For this review, take the finished solid that the model builds, in its own axes (mm). Face numbers are marked on the shaded views. A direction names the side the tool comes from. Coordinates: 2 decimals unless noted, no trailing zeros. Order: outer loops, then holes, each group sorted by start corner. A loop starts at its lowest first (then second) coordinate and runs counter-clockwise, first axis right, second up. Notation, with made-up numbers: M 46,57 L 66,57 A22 cw 66,94 Z; hole C 88.25,-32.5 d2. An arc over 180 degrees is marked long. Use CSV: the item, a comma, the result in double quotes.
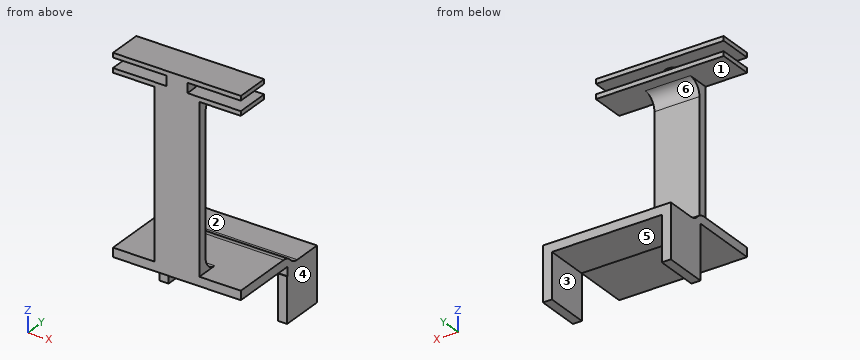
```python
from build123d import *

# Parameters (mm, degrees)
ESQUISSE1_W                = 28.4
ESQUISSE1_H                = 15.1
BOSS_EXTRU_1_DEPTH         = 2
ESQUISSE2_W                = 28.4
ESQUISSE2_H                = 9.6
BOSS_EXTRU_2_DEPTH         = 2
ESQUISSE3_W                = 2
ESQUISSE3_H                = 9.6
ESQUISSE3_H_2              = 9.7
BOSS_EXTRU_3_DEPTH         = 10
ESQUISSE4_W                = 10
ESQUISSE4_H                = 40
BOSS_EXTRU_4_DEPTH         = 2
BOSS_EXTRU_5_DEPTH         = 2.2
ESQUISSE6_W                = 28.4
ESQUISSE6_H                = 7.560696408
BOSS_EXTRU_6_DEPTH         = 1
R_P_TITION_LIN_AIRE1_COUNT = 2
R_P_TITION_LIN_AIRE1_PITCH = 3.2
ESQUISSE7_W                = 2.65
ESQUISSE7_H                = 2.2
ENL_V_MAT_EXTRU_1_DEPTH    = 57.310301011
BOSS_EXTRU_7_DEPTH         = 28.4
CONG_1_R                   = 3


with BuildPart() as part:
    # Esquisse1 → Boss.-Extru.1 (new body)
    with BuildSketch(Plane.XY):
        with Locations((14.2, 7.55)):
            Rectangle(ESQUISSE1_W, ESQUISSE1_H)
    extrude(amount=BOSS_EXTRU_1_DEPTH)

    # Esquisse4 → Boss.-Extru.4 (add)
    with BuildSketch(Plane.XZ):
        with Locations((14.2, 22)):
            Rectangle(ESQUISSE4_W, ESQUISSE4_H)
    extrude(amount=-BOSS_EXTRU_4_DEPTH)

    # Esquisse5 → Boss.-Extru.5 (add)
    with BuildSketch(Plane.XY.offset(42)):
        with BuildLine():
            Line((11.85, 2.5), (11.85, 2))
            Line((11.85, 2), (16.55, 2))
            Line((16.55, 2), (16.55, 2.5))
            ThreePointArc((16.55, 2.5), (14.2, 4.85), (11.85, 2.5))
        make_face()
    extrude(amount=-BOSS_EXTRU_5_DEPTH)

    # Esquisse6 → Boss.-Extru.6 (add)
    with BuildSketch(Plane.XY.offset(42)):
        with Locations((14.2, 3.780348204)):
            Rectangle(ESQUISSE6_W, ESQUISSE6_H)
    boss_extru_6 = extrude(amount=BOSS_EXTRU_6_DEPTH)

    # Répétition linéaire1: Boss.-Extru.6 ×2
    with Locations(*[(0, 0, -i * R_P_TITION_LIN_AIRE1_PITCH) for i in range(1, R_P_TITION_LIN_AIRE1_COUNT)]):
        add(boss_extru_6)

    # Esquisse7 → Enlèv. mat.-Extru.1 (cut, through all)
    with BuildSketch(Plane(origin=(0, 2, 0), x_dir=(1, 0, 0), z_dir=(0, 1, 0))):
        with Locations((17.875, -40.9)):
            Rectangle(ESQUISSE7_W, ESQUISSE7_H)
        with Locations((10.525, -40.9)):
            Rectangle(ESQUISSE7_W, ESQUISSE7_H)
    extrude(amount=-ENL_V_MAT_EXTRU_1_DEPTH, mode=Mode.SUBTRACT)



with BuildPart() as body_2:
    # Esquisse2 → Boss.-Extru.2 (new body)
    with BuildSketch(Plane(origin=(0, 0, 0), x_dir=(-1, 0, 0), z_dir=(0, 0, -1))):
        with Locations((-14.2, 19.9)):
            Rectangle(ESQUISSE2_W, ESQUISSE2_H)
    extrude(amount=BOSS_EXTRU_2_DEPTH)

    # Esquisse3 → Boss.-Extru.3 (add)
    with BuildSketch(Plane(origin=(0, 0, -2), x_dir=(-1, 0, 0), z_dir=(0, 0, -1))):
        with Locations((-1, 19.9)):
            Rectangle(ESQUISSE3_W, ESQUISSE3_H)
        with Locations((-27.4, 19.85)):
            Rectangle(ESQUISSE3_W, ESQUISSE3_H_2)
    extrude(amount=BOSS_EXTRU_3_DEPTH)


with BuildPart() as part_1:
    add(part.part)

    add(body_2.part)  # Boss.-Extru.7 merges body 2
    # Esquisse9 → Boss.-Extru.7 (add)
    with BuildSketch(Plane.ZY):
        Polygon((0, 15.1), (2, 15.1), (0, 17), align=None)
    extrude(amount=-BOSS_EXTRU_7_DEPTH)

    # Congé1
    cong_1_edges = [part_1.edges().sort_by_distance(p)[0] for p in [
        (14.2, 17, 0),
        (14.2, 15.1, 2),
        (14.2, 2, 2),
        (14.2, 2, 38.8),
    ]]
    fillet(cong_1_edges, radius=CONG_1_R)


solid = part_1.part
```
Item 1: For the marked faces 1, 2 and 3, list the 3-axis set-ups (+Z, -Z, +X, -X, +Y, -Y) from which the entire face can be reached by the end or side of a thin tool; tool diameter is ignored.
Solutions:
face 1,"+Y"
face 2,"+Z, +X, -X, +Y"
face 3,"-Z, +Y, -Y"
Item 2: To check wall thickness, follow line 1 along Z through (x, y) = (6, 2.5); line 2 along Y through (x, z) = (18.25, 19); line 3 along X through (y, z) = (16.5, -5.5). State the ranges of each line that lie inside material, in increasing order. Write a range as [from, to].
Solutions:
line 1,"[0, 2], [38.8, 39.8], [42, 43]"
line 2,"[0, 2]"
line 3,"[0, 2], [26.4, 28.4]"
Item 3: Add section A-A on x = 25. State the section outline as (y, z) points.
Solutions:
outline,"M 0,0 L 15.1,0 L 15.1,-2 L 24.7,-2 L 24.7,0 L 18.29,0 A3 cw 16.11,0.93 L 15.99,1.07 A3 ccw 13.81,2 L 0,2 Z; M 0,38.8 L 7.56,38.8 L 7.56,39.8 L 0,39.8 Z; M 0,42 L 7.56,42 L 7.56,43 L 0,43 Z"
Item 4: Add section D-D on z = 16. State the section outline as (x, y) points, and give its area (3 significant figures).
Solutions:
outline,"M 9.2,0 L 19.2,0 L 19.2,2 L 9.2,2 Z"
area,"20.0 mm^2"
Item 5: Add section B-B on y = 3.75. State the section outline as (x, z) points.
Solutions:
outline,"M 0,0 L 28.4,0 L 28.4,2 L 19.2,2 L 19.2,2.27 L 9.2,2.27 L 9.2,2 L 0,2 Z; M 0,38.8 L 9.2,38.8 L 9.2,38.53 L 19.2,38.53 L 19.2,38.8 L 28.4,38.8 L 28.4,39.8 L 16.19,39.8 L 16.19,42 L 28.4,42 L 28.4,43 L 0,43 L 0,42 L 12.21,42 L 12.21,39.8 L 0,39.8 Z"
Item 6: Draft analysis for pull direction Z (two halves, no side actions). For the marked faces 4, 5 and 6, state which applies: released by +Z, released by -Z, zero draft, split by the parting line, or undercut.
Solutions:
face 4,"zero draft"
face 5,"released by -Z"
face 6,"undercut"
Item 7: Add section C-C on x = 14.2. State the section outline as (y, z) points.
Solutions:
outline,"M 0,0 L 15.1,0 L 15.1,-2 L 24.7,-2 L 24.7,0 L 18.29,0 A3 cw 16.11,0.93 L 15.99,1.07 A3 ccw 13.81,2 L 5,2 A3 cw 2,5 L 2,35.8 A3 cw 5,38.8 L 7.56,38.8 L 7.56,39.8 L 4.85,39.8 L 4.85,42 L 7.56,42 L 7.56,43 L 0,43 Z"
Item 8: Clearance check with flat-ended pins moving along their axes: pin 1 Ø1 at (x, y) = (8, 18) entering from -Z; pin 2 Ø1.5 at (y, z) = (1.5, 16) entering from -X; pin 3 Ø12 at (x, y) = (14.5, 6.5) entering from -Z. State where each tip first meets the part, or that it passes through.
Solutions:
pin 1,"z = -2"
pin 2,"x = 9.2"
pin 3,"z = 0"
